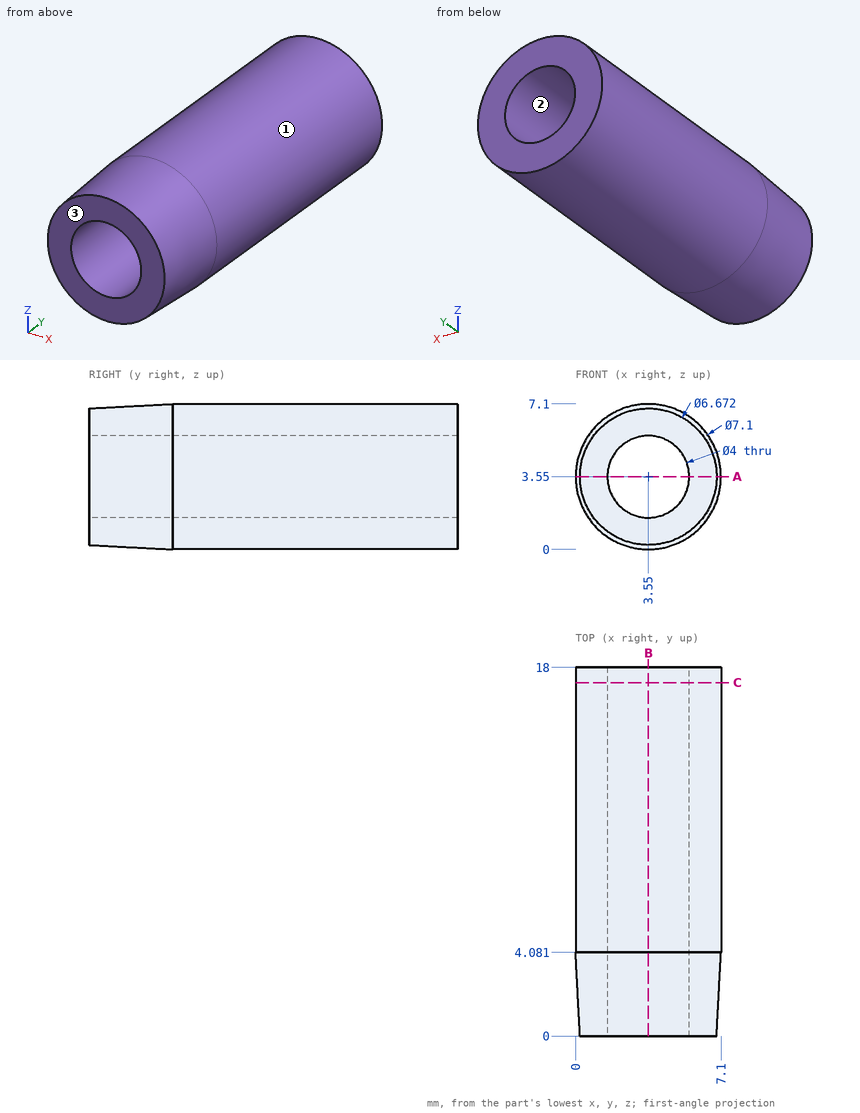
Print and shaded views of the part. All mm, measured from the part's lowest x, y and z. Coordinates: 2 decimals unless noted, no trailing zeros. Order: outer loops, then holes, each group sorted by start corner. A loop starts at its lowest first (then second) coordinate and runs counter-clockwise, first axis right, second up. Notation, with made-up numbers: (16.25, -10) -> (52.25, -10) arc R16 ccw to (52.25, 19) -> close; hole circle Ø9 at (-27, 28.25). An arc over 180 degrees is marked (long way). Use one line per item in the form item = value. Start each with the question number.
1) Band-saw the part on C-C on y = 17.25. Give the cut face in (x, z).
2) Pull direction X, two halves, no side cores. Call the marked faces 1, 2 and 3: +X half, -X half, draft (parallel to the pull), parting line (faces both ways), or undercut.
3) Drop flat-ended pins along their axis: pin 1 (1 mm diameter, centred on x = 5, y = 11.5, fed in from -Z); pin 2 (1.5 mm diameter, centred on y = 10.5, z = 1, fed in from -X). Give the stop position or say it passes through.
4) Band-saw the part on A-A on z = 3.55. Give the cut face in (x, y).
5) Drill centre lines: L1, parallel to Z at x = 3.55, y = 7.75; L2, parallel to Z at x = 4.5, y = 13.75; L3, parallel to X at y = 10.5, z = 3.75. Where is each one in solid material? Low to high. Write a range as [from, to].
6) Band-saw the part on B-B on x = 3.55. Give the cut face in (y, z).
Entries:
q1.outline = circle Ø7.1 at (3.55, 3.55); hole circle Ø4 at (3.55, 3.55)
q2.face_1 = parting line
q2.face_2 = undercut
q2.face_3 = draft
q3.pin_1 = 0.13
q3.pin_2 = 0.49
q4.outline = (0, 4.08) -> (0.21, 0) -> (1.55, 0) -> (1.55, 18) -> (0, 18) -> close; (5.55, 0) -> (6.89, 0) -> (7.1, 4.08) -> (7.1, 18) -> (5.55, 18) -> close
q5.L1 = [0, 1.55], [5.55, 7.1]
q5.L2 = [0.13, 1.79], [5.31, 6.97]
q5.L3 = [0.01, 1.56], [5.54, 7.09]
q6.outline = (0, 0.21) -> (4.08, 0) -> (18, 0) -> (18, 1.55) -> (0, 1.55) -> close; (0, 5.55) -> (18, 5.55) -> (18, 7.1) -> (4.08, 7.1) -> (0, 6.89) -> close
